Check sheet for the modelled part. Datum: model origin and axes. Units: mm. A direction names the side the tool comes from. Give positions to 0.01 mm unless a question says otherwise; leave off trailing zeros. Write each loop counter-clockwise with the first axis right and the second up, starting at its lowest first coordinate (ties: lowest second). Pieces come first, ordered by that corner, then holes. Notation, with made-up numbers: M 24,-5.5 L 37,-5.5 A19 ccw 37,23.5 Z; hole C 30.5,-31.5 d6. An arc over 180 degrees is marked long. One line per item, written item: value. Start each with the question number.
from build123d import *

# Parameters (mm, degrees)
F0_W      = 116.4809949696
F0_H      = 83.6853701621
F1_DEPTH  = 256.032
F2_W      = 24.6532578021
F2_H      = 22.1879333258
F3_DEPTH  = 146.05
F5_DEPTH  = 24.384
F6_R      = 33.7265634664
F9_R      = 50.7557548826
F10_DEPTH = 3.556
F11_W     = 29.1482340544
F11_H     = 8.6365044117
F12_DEPTH = 5.588
F14_DEPTH = 8.5344
F15_W     = 46.036280226
F15_H     = 24.5366059244
F16_DEPTH = 0.762
F17_W     = 46.036280226
F17_H     = 8.0885775387
F18_DEPTH = 1.778
F19_W     = 46.036280226
F19_H     = 7.2142649442
F20_DEPTH = 1.778
F21_W     = 46.036280226
F21_H     = 7.3891170323
F22_DEPTH = 1.778


# Not quite as in the source:
# - the program builds the solid bodies; features that only make, move or delete a surface that nothing else refers to are left out


with BuildPart() as f1:
    # F0 (on Front) → F1 (new body)
    with BuildSketch(Plane.XZ):
        with Locations((23.220455274, -23.1154998764)):
            Rectangle(F0_W, F0_H)
    extrude(amount=-F1_DEPTH)

    # F2 (on face) → F3 (join)
    with BuildSketch(Plane.XY.offset(18.7271852046)):
        with Locations((21.9421936199, 143.5368284583)):
            Rectangle(F2_W, F2_H)
    extrude(amount=F3_DEPTH)

    # F4 (on face) → F5 (join)
    with BuildSketch(Plane(origin=(9.6155647188, 0, 0), x_dir=(0, -1, 0), z_dir=(-1, 0, 0))):
        Polygon((-132.4428617954, 247.5340366364), (-154.6307951212, 164.7771852046), (-132.4428617954, 164.7771852046), (-114.2979115248, 238.0615323782), (-34.0974070132, 290.4760241508), (77.0465955138, 309.4210326672), (149.6690958738, 299.3170320988), (149.6690958738, 318.8935518265), (77.0465955138, 330.8920264244), (-39.1494072974, 311.315536499), align=None)
    extrude(amount=-F5_DEPTH)

    # F6
    f6_edges = [f1.edges().sort_by_distance(p)[0] for p in [
        (-35.020042, 128.016, 18.727185),
        (81.460953, 128.016, 18.727185),
        (-35.020042, 128.016, -64.958185),
        (81.460953, 128.016, -64.958185),
    ]]
    fillet(f6_edges, radius=F6_R)

    # F9 (on face) → F10 (join)
    with BuildSketch(Plane.XZ.offset(149.6690958738)):
        with Locations((21.8075647188, 309.1052919626)):
            Circle(F9_R)
    extrude(amount=F10_DEPTH)

    # F11 (on face) → F12 (join)
    with BuildSketch(Plane.XZ):
        with Locations((22.6024175063, -50.9459078312)):
            Rectangle(F11_W, F11_H)
    extrude(amount=F12_DEPTH)

    # F13 (on face) → F14 (join)
    with BuildSketch(Plane(origin=(0, 0, -55.264160037), x_dir=(1, 0, 0), z_dir=(0, 0, -1))):
        Polygon((32.6312892139, 11.0850147903), (22.6024175063, 5.588), (32.6312892139, 5.588), align=None)
        Polygon((10.6680989265, 11.0850147903), (10.6680989265, 5.588), (22.6024175063, 5.588), align=None)
    extrude(amount=-F14_DEPTH)

    # F15 (on face) → F16 (join)
    with BuildSketch(Plane.XZ):
        with Locations((25.6846474949, -12.2683029622)):
            Rectangle(F15_W, F15_H)
    extrude(amount=F16_DEPTH)

    # F17 (on face) → F18 (join)
    with BuildSketch(Plane.XZ.offset(0.762)):
        with Locations((25.6846474949, -4.0442887694)):
            Rectangle(F17_W, F17_H)
    extrude(amount=F18_DEPTH)

    # F19 (on face) → F20 (join)
    with BuildSketch(Plane.XZ.offset(0.762)):
        with Locations((25.6846474949, -12.7054592595)):
            Rectangle(F19_W, F19_H)
    extrude(amount=F20_DEPTH)

    # F21 (on face) → F22 (join)
    with BuildSketch(Plane.XZ.offset(0.762)):
        with Locations((25.6846474949, -20.8420474082)):
            Rectangle(F21_W, F21_H)
    extrude(amount=F22_DEPTH)


solid = f1.part
1) Gauge pin test, flat ends, axial feed: pin 1 (2 mm diameter, centred on x = 29, y = -1.5, fed in from -Z); pin 2 (14.5 mm diameter, centred on x = 32, y = 191.5, fed in from +Z); pin 3 (2 mm diameter, centred on x = 28.5, y = -0.5, fed in from -Z); pin 4 (24.5 mm diameter, centred on y = 138.5, z = 112.5, fed in from +X). Record the tip position at first contact, or that the pin passes through.
2) Material ranges on L1, parallel to Z at x = 7, y = 191.5; L2, parallel to Z at x = 10, y = 13; L3, parallel to Y at x = -22, z = 328, recorded low to high. Write a range as from..to.
3) Cross-section at A-A (x = 63.5). Record the boundary of the cut face in (y, z).
4) Draft check along Z on faces 5 (the flat face through (22, 0, -32)), 6 (the flat face through (22, -4, -55.264)), 7 (the flat face through (21, -153.225, 310)). Enter one of: released by +Z, released by -Z, zero draft, split by the parting line, or undercut.
5) Cross-section at B-B (y = 80.5). Record the boundary of the cut face in (x, z), plus the area to 3 significant figures.
6) Cross-section at C-C (y = 199.5). Record the boundary of the cut face in (x, z), plus the area to 3 significant figures.
7) Cross-section at D-D (z = 144.5). Record the boundary of the cut face in (x, y), plus the area to 3 significant figures.
8) Tool access check on faces 1 (the flat face through (21.6, 123.5, 200.9)), 2 (the flat face through (34, 37, 291)), 3 (the flat face through (34.269, 143, 91)), 4 (the flat face through (21.64, -113.87, 324.81)). Record the directions out of +Z, -Z, +X, -X, +Y, -Y that give a thin tool (end or side, any length) a straight path to the whole face; none if there is none.
Data:
1. pin 1: stops at z = -55.26
1. pin 2: stops at z = 18.73
1. pin 3: stops at z = -64.96
1. pin 4: stops at x = 34.27
2. L1: z = -64.96..18.73
2. L2: z = -64.96..18.73, 294.07..315.72
2. L3: y = -153.23..-149.67
3. outline: M -153.23,280.16 L -149.67,280.16 L -149.67,338.05 L -153.23,338.05 Z; M 0,-61.05 L 256.03,-61.05 L 256.03,14.82 L 0,14.82 Z
4. face 5: undercut
4. face 6: released by -Z
4. face 7: zero draft
5. outline: M -35.02,-31.23 A33.73 ccw -1.29,-64.96 L 47.73,-64.96 A33.73 ccw 81.46,-31.23 L 81.46,-15 A33.73 ccw 47.73,18.73 L -1.29,18.73 A33.73 ccw -35.02,-15 Z; M 9.62,260.15 L 34,260.15 L 34,283.05 L 9.62,283.05 Z
5. area: 9,330 mm2
6. outline: M -35.02,-31.23 A33.73 ccw -1.29,-64.96 L 47.73,-64.96 A33.73 ccw 81.46,-31.23 L 81.46,-15 A33.73 ccw 47.73,18.73 L -1.29,18.73 A33.73 ccw -35.02,-15 Z
6. area: 8,770 mm2
7. outline: M 9.62,132.44 L 34.27,132.44 L 34.27,154.63 L 9.62,154.63 Z
7. area: 547 mm2
8. face 1: +X, -X, -Y
8. face 2: +Z, +X, +Y
8. face 3: +Z, +X, +Y, -Y
8. face 4: +Z, +X, -X
